Here's how the part is built. I have some questions about the finished solid (model axes, mm). Face numbers are marked on the shaded views. A direction names the side the tool comes from. Coordinates: 2 decimals unless noted, no trailing zeros. Write each loop counter-clockwise with the first axis right and the second up, starting at its lowest first coordinate (ties: lowest second). Pieces come first, ordered by that corner, then holes. Notation, with made-up numbers: M -10.75,64 L 7.25,64 A29 cw 7.25,95 Z; hole C -33,-19.5 d5. An arc over 180 degrees is marked long. Use one line per item in the form item = value. Start each with the question number.
1. I'm going to push flat-ended pins straight in: pin 1 Ø7 at (x, z) = (0, -9) entering from +Y; pin 2 Ø2 at (y, z) = (6.5, 8) entering from -X; pin 3 Ø1 at (x, y) = (3, 10.5) entering from -Z; pin 4 Ø1 at (y, z) = (5.5, -5.5) entering from +X. Where does each tip first touch, or does it pass through?
2. I want a section at C-C, the plane x = -12. List the corners of the cut face in (y, z) for me.
3. I want a section at D-D, the plane z = 9. List the corners of the cut face in (x, y) for me.
4. I want a section at A-A, the plane x = 0. List the corners of the cut face in (y, z) for me.
5. Thinking about a two-plate mould opening in Z: for the marked faces 4, 5 and 6, which applies, released by +Z, released by -Z, zero draft, split by the parting line, or undercut?
6. On a 3-axis mill with a long thin cutter (end or side, diameter ignored), from which of +Z, -Z, +X, -X, +Y, -Y can I reach the whole of each face in a straight line? I mean the marked faces 1, 2 and 3. Say none if no direction works.
7. I want a section at B-B, the plane y = 7. List the corners of the cut face in (x, z) for me, plus the area to 3 significant figures.
8. Please list where these lines run through material, in increasing order: line 1 along Z through (x, y) = (-5.75, 4.25); line 2 along Z through (x, y) = (-1.25, 8); line 3 along Z through (x, y) = (-0.75, 5). Write a range as [from, to].
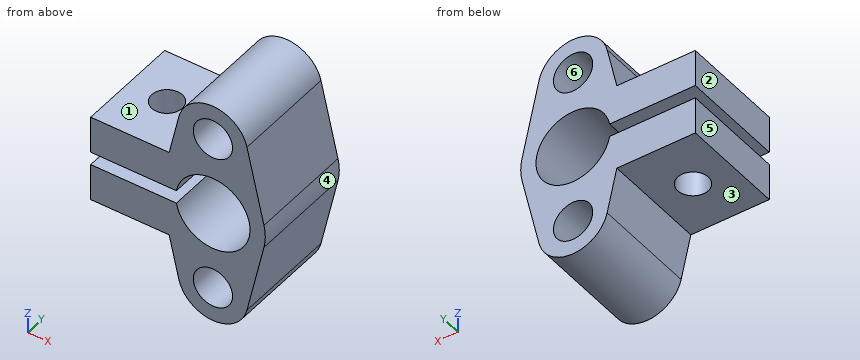
Autodesk Inventor part; units mm, degrees
ref_plane "YZ Plane" through (0, 0, 0) normal (1, 0, 0) x (0, 1, 0)
ref_plane "XZ Plane" through (0, 0, 0) normal (0, 1, 0) x (-1, 0, 0)
ref_plane "XY Plane" through (0, 0, 0) normal (0, 0, 1) x (1, 0, 0)
sketch "Sketch1" plane through (0, 0, 0) normal (0, 1, 0) x (-1, 0, 0)
  circle A0 centre (0, 0) radius 4.25
  circle A1 centre (0, 0) radius 6
  line L0 (14, 5) -> (14, -5)
  line L1 (4.1833, 0.75) -> (14, 0.75)
  line L2 (14, 0.75) -> (14, -0.75)
  line L3 (14, -0.75) -> (4.1833, -0.75)
  circle A2 centre (0, 9) radius 2.25
  circle A3 centre (0, -9) radius 2.25
  circle A4 centre (0, 9) radius 4
  circle A5 centre (0, -9) radius 4
  line L4 (3.9, 9.8889) -> (5.85, 1.3333)
  line L5 (-3.9, 9.8889) -> (-5.85, 1.3333)
  line L6 (5.85, -1.3333) -> (3.9, -9.8889)
  line L7 (-5.85, -1.3333) -> (-3.9, -9.8889)
  line L8 (3.3166, -5) -> (14, -5)
  line L9 (14, 5) -> (3.3166, 5)
  line L10 (18, 0) -> (-10, 0)
  point P0 (14, 0)
  point P1 (14, -0.75)
  point P2 (14, 0.75)
  point P3 (5.0143, -5)
  point P4 (5.0143, 5)
  point P5 (5.9529, -0.75)
  point P6 (6, 0)
  point P7 (14, 0)
  dimension "d0" = 8.5
  dimension "d1" = 12
  dimension "d2" = 10
  dimension "d3" = 14
  dimension "d4" = 1.5
  dimension "d5" = 14
  dimension "d6" = 4.5
  dimension "d7" = 4.5
  dimension "d8" = 18
  dimension "d9" = 9
  dimension "d10" = 8
  dimension "d11" = 8
  dimension "d30" = 5
extrude "Extrusion1" add sketch "Sketch1" along normal blind 12 contours A0 L10 A1 A4 L1 | L3 A1 A5 L10 A0 | A1 L4 L9 L0 L1 | L3 L0 L8 L6 A1 | A1 L9 L4 | L6 L8 A1 | L5 A4 A1 | A1 A5 L7 | A1 A4 L4 L9 | L8 L6 A5 A1 | A4 A1 | A1 A4 | A5 A1 | A1 A5
sketch "Sketch4" plane through (-14, 0, 5) normal (0, 0, 1) x (1, 0, 0)
  line L0 (0, 0) -> (8.9857, 0)
  line L1 (0, 12) -> (8.9857, 12)
  point P0 (14, 0)
  point P1 (4.5, 6)
  dimension "d31" = 6
  dimension "d32" = 6
  dimension "d33" = 4.5
hole "Hole1" at (-9.5, 6, 5) direction (0, 0, -1) diameter 3.5 depth 10
equation "\"d12\" = d1"
properties part number "Kep_Truc"
Answer list:
q1.pin_1 = 12
q1.pin_2 = -4.56
q1.pin_3 = -12.12
q1.pin_4 = 5.01
q2.outline = M 0,-5 L 12,-5 L 12,-0.75 L 0,-0.75 Z; M 0,0.75 L 12,0.75 L 12,5 L 0,5 Z
q3.outline = M -4.1,0 L -2.25,0 L -2.25,12 L -4.1,12 Z; M 2.25,0 L 4.1,0 L 4.1,12 L 2.25,12 Z
q4.outline = M 0,-13 L 12,-13 L 12,-11.25 L 0,-11.25 Z; M 0,-6.75 L 12,-6.75 L 12,-4.25 L 0,-4.25 Z; M 0,4.25 L 12,4.25 L 12,6.75 L 0,6.75 Z; M 0,11.25 L 12,11.25 L 12,13 L 0,13 Z
q5.face_4 = split by the parting line
q5.face_5 = zero draft
q5.face_6 = undercut
q6.face_1 = +Z, -X, +Y, -Y
q6.face_2 = +Z, -Z, -X, +Y, -Y
q6.face_3 = -Z, -X, +Y, -Y
q7.outline = M -14,-5 L -10.94,-5 L -10.94,-0.75 L -14,-0.75 Z; M -14,0.75 L -10.94,0.75 L -10.94,5 L -14,5 Z; M -8.06,-5 L -5.01,-5 L -3.9,-9.89 A4 ccw 3.9,-9.89 L 5.85,-1.33 A6 ccw 5.85,1.33 L 3.9,9.89 A4 ccw -3.9,9.89 L -5.01,5 L -8.06,5 L -8.06,0.75 L -4.18,0.75 A4.25 cw long -4.18,-0.75 L -8.06,-0.75 Z; hole C 0,-9 d4.5; hole C 0,9 d4.5
q7.area = 191 mm²
q8.line_1 = [-5, -0.75], [0.75, 5]
q8.line_2 = [-12.8, -10.87], [-7.13, -4.06], [4.06, 7.13], [10.87, 12.8]
q8.line_3 = [-12.93, -11.12], [-6.88, -4.18], [4.18, 6.88], [11.12, 12.93]
